from build123d import *

# Parameters (mm, degrees)
SKETCH1_R           = 2.5
BOSS_EXTRUDE2_DEPTH = 4.5
SKETCH1_3_R         = 3.5
SKETCH1_3_R_2       = 2.5
BOSS_EXTRUDE3_DEPTH = 4.5
SKETCH1_4_R         = 3.5
SKETCH1_4_R_2       = 2.5
CUT_EXTRUDE1_DEPTH  = 2
SKETCH2_R           = 2.05
CUT_EXTRUDE2_DEPTH  = 1.8


with BuildPart() as part:
    # Sketch1 → Boss-Extrude2 (new body)
    with BuildSketch(Plane(origin=(0, 0, 0), x_dir=(1, 0, 0), z_dir=(0, 1, 0))):
        with Locations(Location((0, 0, 0), (0, 0, 270))):
            Circle(SKETCH1_R)
    extrude(amount=BOSS_EXTRUDE2_DEPTH)

    # Sketch1<3> → Boss-Extrude3 (add)
    with BuildSketch(Plane(origin=(0, 0, 0), x_dir=(1, 0, 0), z_dir=(0, 1, 0))):
        with Locations(Location((0, 0, 0), (0, 0, 270))):
            Circle(SKETCH1_3_R)
        Circle(SKETCH1_3_R_2, mode=Mode.SUBTRACT)
    extrude(amount=BOSS_EXTRUDE3_DEPTH)

    # Sketch1<4> → Cut-Extrude1 (cut)
    with BuildSketch(Plane(origin=(0, 0, 0), x_dir=(1, 0, 0), z_dir=(0, 1, 0))):
        with Locations(Location((0, 0, 0), (0, 0, 270))):
            Circle(SKETCH1_4_R)
        with Locations(Location((0, 0, 0), (0, 0, 270))):
            Circle(SKETCH1_4_R_2, mode=Mode.SUBTRACT)
    extrude(amount=CUT_EXTRUDE1_DEPTH, mode=Mode.SUBTRACT)

    # Sketch2 → Cut-Extrude2 (cut)
    with BuildSketch(Plane(origin=(0, 4.5, 0), x_dir=(1, 0, 0), z_dir=(0, 1, 0))):
        with Locations(Location((0, 0, 0), (0, 0, 270))):
            Circle(SKETCH2_R)
    extrude(amount=-CUT_EXTRUDE2_DEPTH, mode=Mode.SUBTRACT)


solid = part.part
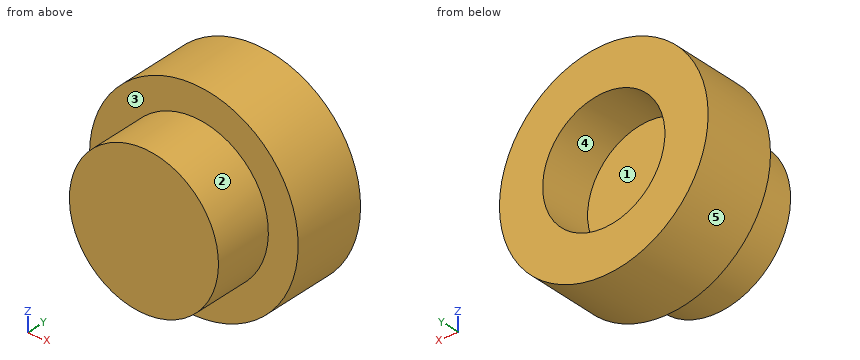
Input: part model. Units: mm. Frame: model coordinates. Face numbers are marked on the shaded views. A direction names the side the tool comes from. Give positions to 0.01 mm unless a question says otherwise; leave off trailing zeros. Order: outer loops, then holes, each group sorted by start corner. A loop starts at its lowest first (then second) coordinate and runs counter-clockwise, first axis right, second up. Notation, with made-up numbers: (52, 38.5) - (72, 38.5) arc R13 ccw to (72, 43.5) - close; hole circle Ø11 at (-3.75, 27). An arc over 180 degrees is marked (long way). Answer as a JSON object with one key per item and string values. Group by question number.
Q1. Cut plane A-A, the plane z = 0. Output: boundary loops of the cut face in (x, y).
Q2. Set-up query: the marked faces 4 and 5. Return all of +Z, -Z, +X, -X, +Y, -Y with unobstructed straight access to the full face (end or side cutting, diameter ignored); none if empty.
Q3. Cut plane D-D, the plane y = 1.15. Output: boundary loops of the cut face in (x, z).
Q4. Mould query, pull axis Z, two halves, no side actions, for the marked faces 1, 2 and 3. Classes: pulls with the +Z half, pulls with the -Z half, needs draft (parallel to the pull), parting line crosses it, or undercut.
Q5. Cut plane C-C, the plane x = 0. Output: boundary loops of the cut face in (y, z), then the cut area to 3 significant figures.
Q6. First-contact query: pin 1 Ø1 at (y, z) = (4, 1.5) entering from +X; pin 2 Ø1.2 at (x, z) = (0.5, 0) entering from +Y. Flat tips, straight axial feed; report the tip coordinate or a pass-through.
Q7. Line query: probe 1 along X at (y, z) = (3.6, 0); probe 2 along Y at (x, z) = (-2.5, -1); probe 3 along Y at (x, z) = (1, -0.5). Output: solid intervals per line, ascending.
Q8. Cut plane B-B, the plane y = 3.2. Output: boundary loops of the cut face in (x, z), then the cut area to 3 significant figures.
Results:
{
 "1": {"outline": "(-3.5, 2) - (-2.5, 2) - (-2.5, 0) - (2.5, 0) - (2.5, 2) - (3.5, 2) - (3.5, 4.5) - (2.05, 4.5) - (2.05, 2.7) - (-2.05, 2.7) - (-2.05, 4.5) - (-3.5, 4.5) - close"},
 "2": {"face 4": "+Y", "face 5": "+Y, -Y"},
 "3": {"outline": "circle Ø5 at (0, 0)"},
 "4": {"face 1": "undercut", "face 2": "parting line crosses it", "face 3": "needs draft"},
 "5": {"outline": "(0, -2.5) - (2, -2.5) - (2, -3.5) - (4.5, -3.5) - (4.5, -2.05) - (2.7, -2.05) - (2.7, 2.05) - (4.5, 2.05) - (4.5, 3.5) - (2, 3.5) - (2, 2.5) - (0, 2.5) - close", "area": "20.1 mm^2"},
 "6": {"pin 1": "x = 3.35", "pin 2": "y = 2.7"},
 "7": {"probe 1": "-3.5 to -2.05, 2.05 to 3.5", "probe 2": "2 to 4.5", "probe 3": "0 to 2.7"},
 "8": {"outline": "circle Ø7 at (0, 0); hole circle Ø4.1 at (0, 0)", "area": "25.3 mm^2"}
}
